Geometry check sheet. Reference: the model listing, model coordinates, mm. A direction names the side the tool comes from. Coordinates: 2 decimals unless noted, no trailing zeros. Write each loop counter-clockwise with the first axis right and the second up, starting at its lowest first coordinate (ties: lowest second). Pieces come first, ordered by that corner, then holes. Notation, with made-up numbers: (35, 10.25) -> (55, 10.25) arc R14 cw to (55, 31.25) -> close; hole circle Ø8 at (-37, 35.5). An arc over 180 degrees is marked (long way). Use a Markdown table: item, result.
```python
from build123d import *

# Parameters (mm, degrees)
F1_DEPTH = 6
F2_R     = 4.7625
F3_DEPTH = 25
F4_R     = 4.7625
F5_DEPTH = 3
F6_SIZE  = 1.2


with BuildPart() as f1:
    # F0 (on Top) → F1 (new body)
    with BuildSketch(Plane.XY):
        with BuildLine():
            ThreePointArc((-30.2148338807, -47.1672770381), (-27.2859016925, -54.23834485), (-20.2148338807, -57.1672770381))
            Line((-20.2148338807, -57.1672770381), (59.7851661193, -57.1672770381))
            ThreePointArc((59.7851661193, -57.1672770381), (66.8562339312, -54.23834485), (69.7851661193, -47.1672770381))
            Line((69.7851661193, -47.1672770381), (69.7851661193, 42.8327229619))
            ThreePointArc((69.7851661193, 42.8327229619), (66.8562339312, 49.9037907738), (59.7851661193, 52.8327229619))
            Line((59.7851661193, 52.8327229619), (-20.2148338807, 52.8327229619))
            ThreePointArc((-20.2148338807, 52.8327229619), (-27.2859016925, 49.9037907738), (-30.2148338807, 42.8327229619))
            Line((-30.2148338807, 42.8327229619), (-30.2148338807, -47.1672770381))
        make_face()
    extrude(amount=F1_DEPTH)

    # F2 (on face) → F3 (cut)
    with BuildSketch(Plane.XY.offset(6)):
        with Locations((19.7851661193, -2.1672770381)):
            Circle(F2_R)
    extrude(amount=-F3_DEPTH, mode=Mode.SUBTRACT)

    # F4 (on face) → F5 (cut)
    with BuildSketch(Plane(origin=(0, 0, 0), x_dir=(1, 0, 0), z_dir=(0, 0, -1))):
        Polygon((26.9352661193, -1.9608351216), (26.9352661193, 6.2953891978), (19.7851661193, 10.4235013576), (12.6350661193, 6.2953891978), (12.6350661193, -1.9608351216), (19.7851661193, -6.0889472814), align=None)
        with Locations((19.7851661193, 2.1672770381)):
            Circle(F4_R, mode=Mode.SUBTRACT)
    extrude(amount=-F5_DEPTH, mode=Mode.SUBTRACT)

    # F6
    f6_edges = [f1.edges().sort_by_distance(p)[0] for p in [
        (-27.285902, 49.903791, 6),
        (19.785166, 52.832723, 6),
        (-30.214834, -2.167277, 6),
        (66.856234, 49.903791, 6),
        (-27.285902, -54.238345, 6),
        (69.785166, -2.167277, 6),
        (19.785166, -57.167277, 6),
        (66.856234, -54.238345, 6),
        (15.022666, -2.167277, 6),
    ]]
    chamfer(f6_edges, length=F6_SIZE)


solid = f1.part
```
Item 1: Mould release check, pull along X, two halves, no side actions. Record for faces 3 (the flat face through (8, -1, 6)), 4 (the cylindrical face through (-27.21, 49.98, 2.37)), 5 (the flat face through (12.635, -2, 1)): +X half, -X half, draft (parallel to the pull), parting line (faces both ways), or undercut.
Answer block:
| item | result |
|---|---|
| face 3 | draft |
| face 4 | -X half |
| face 5 | undercut |
Item 2: Thickness scan on L1, parallel to Y at x = 24, z = 0.8; L2, parallel to Y at x = 28.5, z = 5.35; L3, parallel to Y at x = 38, z = 5. Record the ranges inside material, lowest first. Write a range as [from, to].
Answer block:
| item | result |
|---|---|
| L1 | y = [-57.17, -7.99], [3.66, 52.83] |
| L2 | y = [-56.62, 52.28] |
| L3 | y = [-56.97, 52.63] |
Item 3: Depth check by flat-ended pin: P1, Ø4.5, axis at x = 21.5, y = -2.5, coming from the -Z side. Enter the tip coordinate at first touch or a pass-through.
Answer block:
| item | result |
|---|---|
| P1 | passes through |
Item 4: Section check A-A on z = 2.05. Record the boundary of the cut face in (x, y), then the cut area to 3 significant figures.
Answer block:
| item | result |
|---|---|
| outline | (-30.21, -47.17) arc R10 ccw to (-20.21, -57.17) -> (59.79, -57.17) arc R10 ccw to (69.79, -47.17) -> (69.79, 42.83) arc R10 ccw to (59.79, 52.83) -> (-20.21, 52.83) arc R10 ccw to (-30.21, 42.83) -> close; hole (12.64, -6.3) -> (19.79, -10.42) -> (26.94, -6.3) -> (26.94, 1.96) -> (19.79, 6.09) -> (12.64, 1.96) -> close |
| area | 10,700 mm^2 |
Item 5: Tool access check on faces 1 (the conical face through (66.225, 49.132, 5.792)), 2 (the flat face through (23.41, -8.33, 1.48)). Record the directions out of +Z, -Z, +X, -X, +Y, -Y that give a thin tool (end or side, any length) a straight path to the whole face; none if there is none.
Answer block:
| item | result |
|---|---|
| face 1 | +Z, +X, +Y |
| face 2 | -Z |
